Design review of the part built by this model. Coordinates are the model's own, in mm. Face numbers are marked on the shaded views. A direction names the side the tool comes from. Round coordinates to 2 decimals unless told otherwise and drop trailing zeros. Write each loop counter-clockwise with the first axis right and the second up, starting at its lowest first coordinate (ties: lowest second). Pieces come first, ordered by that corner, then holes. Notation, with made-up numbers: (22, -33.5) -> (59, -33.5) arc R23 ccw to (59, -4.5) -> close; hole circle Ø11 at (33.5, 27). An arc over 180 degrees is marked (long way). Write item = value, one per line. Start each with the question number.
Item 1: Machinability: for the marked faces 1, 2 and 3, which of the approach directions +Z, -Z, +X, -X, +Y, -Y give a long, thin tool a straight path to every point of the face, cutting with its end or side? Answer none if there is none.
Item 2: To check wall thickness, follow L1, parallel to Y at x = 51.5, z = 28; L2, parallel to X at y = -23.25, z = 20; L3, parallel to Y at x = 40, z = 32.5. State the ranges of each line that lie inside material, in increasing order.
Item 3: Add section C-C, the plane z = 6.5. State the section outline as (x, y) points, then the cut area to 3 significant figures.
Item 4: Add section B-B, the plane x = 53. State the section outline as (y, z) points.
Item 5: For pin 1 Ø1 at (x, z) = (16, 28) entering from +Y; pin 2 Ø1.2 at (y, z) = (-17, 34.5) entering from +X; pin 3 Ø1.2 at (x, z) = (30.5, 35) entering from -Y, all flat-tipped, find the tip position at first contact; note any pin that passes through.
Item 6: Add section A-A, the plane y = -15.5. State the section outline as (x, z) points, then the cut area to 3 significant figures.
Item 7: Mouldability with a two-part tool opening along Y and no side actions: class the marked faces 4, 5 and 6 as released by +Y, released by -Y, zero draft, split by the parting line, or undercut.
Item 8: Add section D-D, the plane z = 30. State the section outline as (x, y) points.
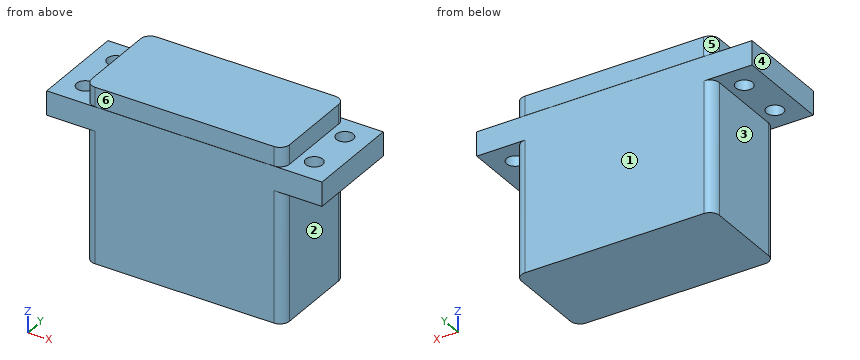
from build123d import *

# Parameters (mm, degrees)
BOSS_EXTRUDE1_DEPTH = 27.21
SKETCH2_W           = 57.1
SKETCH2_H           = 20
BOSS_EXTRUDE2_DEPTH = 5
BOSS_EXTRUDE3_DEPTH = 4
SKETCH4_R           = 1.752596491
CUT_EXTRUDE1_DEPTH  = 5.63


with BuildPart() as part:
    # Sketch1 → Boss-Extrude1 (new body)
    with BuildSketch(Plane.XY):
        with BuildLine():
            Line((9.946325167, -5.324573125), (47.046325167, -5.324573125))
            ThreePointArc((47.046325167, -5.324573125), (48.460538729, -5.910359563), (49.046325167, -7.324573125))
            Line((49.046325167, -7.324573125), (49.046325167, -23.324573125))
            ThreePointArc((49.046325167, -23.324573125), (48.460538729, -24.738786688), (47.046325167, -25.324573125))
            Line((47.046325167, -25.324573125), (9.946325167, -25.324573125))
            ThreePointArc((9.946325167, -25.324573125), (8.532111605, -24.738786688), (7.946325167, -23.324573125))
            Line((7.946325167, -23.324573125), (7.946325167, -7.324573125))
            ThreePointArc((7.946325167, -7.324573125), (8.532111605, -5.910359563), (9.946325167, -5.324573125))
        make_face()
    extrude(amount=BOSS_EXTRUDE1_DEPTH)

    # Sketch2 → Boss-Extrude2 (add)
    with BuildSketch(Plane.XY.offset(27.21)):
        with Locations((28.496325167, -15.324573125)):
            Rectangle(SKETCH2_W, SKETCH2_H)
    extrude(amount=BOSS_EXTRUDE2_DEPTH)

    # Sketch3 → Boss-Extrude3 (add)
    with BuildSketch(Plane.XY.offset(32.21)):
        with BuildLine():
            Line((9.946325167, -5.279301006), (47.046325167, -5.279301006))
            ThreePointArc((47.046325167, -5.279301006), (48.460538729, -5.865087443), (49.046325167, -7.279301006))
            Line((49.046325167, -7.279301006), (49.046325167, -23.279301006))
            ThreePointArc((49.046325167, -23.279301006), (48.460538729, -24.693514568), (47.046325167, -25.279301006))
            Line((47.046325167, -25.279301006), (9.946325167, -25.279301006))
            ThreePointArc((9.946325167, -25.279301006), (8.532111605, -24.693514568), (7.946325167, -23.279301006))
            Line((7.946325167, -23.279301006), (7.946325167, -7.279301006))
            ThreePointArc((7.946325167, -7.279301006), (8.532111605, -5.865087443), (9.946325167, -5.279301006))
        make_face()
    extrude(amount=BOSS_EXTRUDE3_DEPTH)

    # Sketch4 → Cut-Extrude1 (cut)
    with BuildSketch(Plane.XY.offset(32.21)):
        with Locations((4.734760216, -10.324573125)):
            Circle(SKETCH4_R)
        with Locations((4.734760216, -20.324573125)):
            Circle(SKETCH4_R)
        with Locations((52.257890118, -20.324573125)):
            Circle(SKETCH4_R)
        with Locations((52.257890118, -10.324573125)):
            Circle(SKETCH4_R)
    extrude(amount=-CUT_EXTRUDE1_DEPTH, mode=Mode.SUBTRACT)


solid = part.part
Result set:
q1.face_1 = -Z, +X, -X, +Y
q1.face_2 = -Z, +X, +Y, -Y
q1.face_3 = -Z, -X, +Y, -Y
q2.L1 = -25.32 to -21.9, -18.74 to -11.9, -8.74 to -5.32
q2.L2 = 7.95 to 49.05
q2.L3 = -25.28 to -5.28
q3.outline = (7.95, -23.32) arc R2 ccw to (9.95, -25.32) -> (47.05, -25.32) arc R2 ccw to (49.05, -23.32) -> (49.05, -7.32) arc R2 ccw to (47.05, -5.32) -> (9.95, -5.32) arc R2 ccw to (7.95, -7.32) -> close
q3.area = 819 mm²
q4.outline = (-25.32, 27.21) -> (-21.91, 27.21) -> (-21.91, 32.21) -> (-25.32, 32.21) -> close; (-18.74, 27.21) -> (-11.91, 27.21) -> (-11.91, 32.21) -> (-18.74, 32.21) -> close; (-8.74, 27.21) -> (-5.32, 27.21) -> (-5.32, 32.21) -> (-8.74, 32.21) -> close
q5.pin_1 = -5.32
q5.pin_2 = 49.05
q5.pin_3 = -25.28
q6.outline = (-0.05, 27.21) -> (7.95, 27.21) -> (7.95, 0) -> (49.05, 0) -> (49.05, 27.21) -> (57.05, 27.21) -> (57.05, 32.21) -> (49.05, 32.21) -> (49.05, 36.21) -> (7.95, 36.21) -> (7.95, 32.21) -> (-0.05, 32.21) -> close
q6.area = 1,570 mm²
q7.face_4 = zero draft
q7.face_5 = released by +Y
q7.face_6 = released by -Y
q8.outline = (-0.05, -25.32) -> (57.05, -25.32) -> (57.05, -5.32) -> (-0.05, -5.32) -> close; hole circle Ø3.51 at (4.73, -20.32); hole circle Ø3.51 at (4.73, -10.32); hole circle Ø3.51 at (52.26, -20.32); hole circle Ø3.51 at (52.26, -10.32)
